Build history of the part. All positions in model axes, mm. Face numbers are marked on the shaded views. A direction names the side the tool comes from. Coordinates: 2 decimals unless noted, no trailing zeros. Order: outer loops, then holes, each group sorted by start corner. A loop starts at its lowest first (then second) coordinate and runs counter-clockwise, first axis right, second up. Notation, with made-up numbers: (-40, 25) - (-3, 25) arc R35 cw to (-3, 59) - close; hole circle Ø9 at (-26.75, 27). An arc over 180 degrees is marked (long way). Write each question's results on one line, items separated by ' | '. Start each with the question number.
from build123d import *

# Parameters (mm, degrees)
EXTRUDE_1_DEPTH     = 68.52
SKETCH_2_W          = 10.5
SKETCH_2_H          = 1
CUT_EXTRUDE_1_DEPTH = 140.984803019
CHAMFER_1_SIZE      = 1


with BuildPart() as part:
    # 草图1 → 凸台-拉伸1 (new, symmetric)
    with BuildSketch(Plane.XY):
        with BuildLine():
            Line((-16, 0), (16, 0))
            Line((16, 0), (16, 4))
            Line((16, 4), (6.25, 4))
            Line((6.25, 4), (6.25, 8.5))
            Line((6.25, 8.5), (5.25, 8.5))
            Line((5.25, 8.5), (2.651923789, 13))
            ThreePointArc((2.651923789, 13), (0, 23.659743791), (-2.651923789, 13))
            Line((-2.651923789, 13), (-5.25, 8.5))
            Line((-5.25, 8.5), (-6.25, 8.5))
            Line((-6.25, 8.5), (-6.25, 4))
            Line((-6.25, 4), (-16, 4))
            Line((-16, 4), (-16, 0))
        make_face()
    extrude(amount=EXTRUDE_1_DEPTH, both=True)

    # 草图2 → 切除-拉伸1 (cut, through all)
    with BuildSketch(Plane.XY.offset(68.52)):
        with Locations((0, 0.5)):
            Rectangle(SKETCH_2_W, SKETCH_2_H)
    extrude(amount=-CUT_EXTRUDE_1_DEPTH, mode=Mode.SUBTRACT)

    # 倒角1
    chamfer_1_edges = [part.edges().sort_by_distance(p)[0] for p in [
        (5.25, 0, 0),
        (-5.25, 0, 0),
    ]]
    chamfer(chamfer_1_edges, length=CHAMFER_1_SIZE - 0.0001)  # a hair under: the kernel refuses the full size


solid = part.part
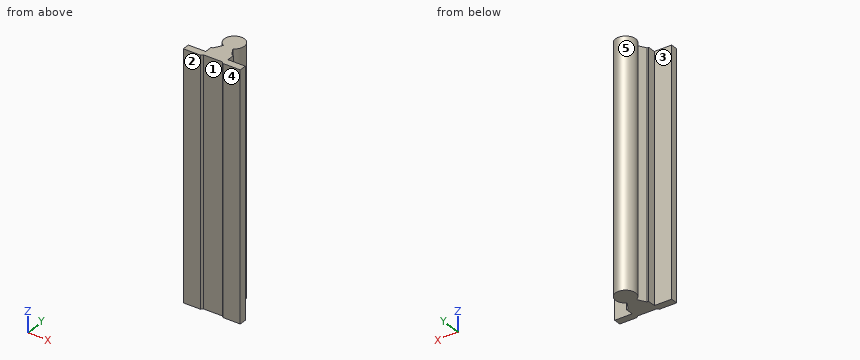
Item 1: Which spindle directions (+Z, -Z, +X, -X, +Y, -Y) get a long thin tool onto all of the face, cutting with end or side? Do the marked faces 1 and 2. Say none if no direction does.
Item 2: Pull direction Y, two halves, no side cores. Call the marked faces 3, 4 and 5: released by +Y, released by -Y, zero draft, split by the parting line, or undercut.
Item 3: Probe probe 1 along X at (y, z) = (6.75, 25.5); probe 2 along Y at (x, z) = (14.5, -44); probe 3 along Y at (x, z) = (5, 1). List the from-to ranges inside material, lowest first.
Item 4: Slice it at C-C (y = 18). Write the cut outline in (x, z).
Item 5: Slice it at B-B (x = 14.5). Write the cut outline in (y, z).
Item 6: Flat gauge pins, fed straight in: P1, Ø5, axis at x = 9.5, z = 0, coming from the +Y side; P2, Ø6, axis at y = 18, z = -29, coming from the +X side; P3, Ø1.5, axis at y = 16, z = -23.5, coming from the +X side. Where does each tip first touch, or does it go through?
Resolved:
1) face 1: +Z, -Z, -Y | face 2: +Z, -Z, +X, -X, -Y
2) face 3: released by +Y | face 4: released by -Y | face 5: undercut
3) probe 1: -6.25 to 6.25 | probe 2: 0 to 4 | probe 3: 1 to 8.93, 15.35 to 20.65
4) outline: (-5.66, -68.52) - (5.66, -68.52) - (5.66, 68.52) - (-5.66, 68.52) - close
5) outline: (0, -68.52) - (4, -68.52) - (4, 68.52) - (0, 68.52) - close
6) P1: y = 4 | P2: x = 5.66 | P3: x = 5.52
